Part model, mm, in its own coordinate system. A direction names the side the tool comes from. Coordinates: 2 decimals unless noted, no trailing zeros. Write each loop counter-clockwise with the first axis right and the second up, starting at its lowest first coordinate (ties: lowest second). Pieces come first, ordered by that corner, then holes. Notation, with made-up numbers: M 38,16 L 79,16 A29 cw 79,46 Z; hole C 44,26.5 d3. An arc over 180 degrees is marked long. Use a Markdown table: item, result. Add a question column.
Q1. Tool access for faces 1 (the flat face through (69, 32, 38)), 2 (the flat face through (69, -38, -32.001)), 3 (the flat face through (4, 30, -6)): list every direction of +Z, -Z, +X, -X, +Y, -Y with a clear straight run to the whole face (end or side of a thin tool).
Q2. Slice it at A-A on y = 15. Write the cut outline in (x, z).
Q3. Slice it at C-C on x = 76. Write the cut outline in (y, z).
Q4. Pin check, flat tips, straight feed: pin 1 Ø4 at (x, y) = (134, -2.5) entering from -Z; pin 2 Ø12 at (x, y) = (73.5, -21.5) entering from +Z. Stop position of each tip, or through.
Q5. Wall check: L1, parallel to Y at x = 2.1, z = -32; L2, parallel to X at y = 37.5, z = -5.5; L3, parallel to Z at x = 38, y = 34.5. Give the ranges that are in metal, low to high. Write a range as from..to.
Q6. Slice it at B-B on z = 0. Write the cut outline in (x, y).
Q7. Mould opens along Z. For faces 4 (the flat face through (69, 36, -34)), 5 (the flat face through (64, -40, -33)), 6 (the flat face through (64, -33, 40)) say: released by +Z, released by -Z, zero draft, split by the parting line, or undercut.
from build123d import *

# Parameters (mm, degrees)
CROQUIS1_W              = 80
CROQUIS1_H              = 80
SALIENTE_EXTRUIR1_DEPTH = 140
CORTAR_EXTRUIR3_DEPTH   = 136
CROQUIS8_R              = 2
CROQUIS8_W              = 55
CROQUIS8_H              = 55
CORTAR_EXTRUIR4_DEPTH   = 136
SALIENTE_EXTRUIR4_DEPTH = 8


with BuildPart() as part:
    # Croquis1 → Saliente-Extruir1 (new body)
    with BuildSketch(Plane.YZ):
        Rectangle(CROQUIS1_W, CROQUIS1_H)
    extrude(amount=SALIENTE_EXTRUIR1_DEPTH)

    # Croquis7 → Cortar-Extruir3 (cut)
    with BuildSketch(Plane.YZ.offset(140)):
        Polygon((-40, 32.000605379), (-36, 32.000605379), (-36, 36), (-32, 36), (-32, 40), (32, 40), (32, 36), (36, 36), (36, 32.000605379), (40, 32.000605379), (40, -32.000605379), (36, -32.000605379), (36, -36), (32, -36), (32, -40), (-32, -40), (-32, -36), (-36, -36), (-36, -32.000605379), (-40, -32.000605379), align=None)
    extrude(amount=-CORTAR_EXTRUIR3_DEPTH, mode=Mode.SUBTRACT)

    # Croquis8 → Cortar-Extruir4 (cut)
    with BuildSketch(Plane.YZ.offset(4)):
        with Locations(Location((-32, 32, 0), (0, 0, 270))):
            Circle(CROQUIS8_R)
        with Locations(Location((-32, -32, 0), (0, 0, 270))):
            Circle(CROQUIS8_R)
        with Locations(Location((32, -32, 0), (0, 0, 270))):
            Circle(CROQUIS8_R)
        with Locations(Location((32, 32, 0), (0, 0, 270))):
            Circle(CROQUIS8_R)
        Rectangle(CROQUIS8_W, CROQUIS8_H)
    extrude(amount=-CORTAR_EXTRUIR4_DEPTH, mode=Mode.SUBTRACT)

    # Croquis9 → Saliente-Extruir4 (add)
    with BuildSketch(Plane.YZ.offset(140)):
        Polygon((32, -40), (40, -40), (40, 40), (-40, 40), (-40, -40), (-32, -40), (-32, 32), (32, 32), align=None)
    extrude(amount=-SALIENTE_EXTRUIR4_DEPTH)


solid = part.part
Recorded:
| question | item | result |
|---|---|---|
| 1 | face 1 | +Z, -Z |
| 1 | face 2 | +Y, -Y |
| 1 | face 3 | none |
| 2 | outline | M 0,-40 L 4,-40 L 4,-27.5 L 0,-27.5 Z; M 0,27.5 L 4,27.5 L 4,40 L 0,40 Z; M 132,32 L 140,32 L 140,40 L 132,40 Z |
| 3 | outline | M -40,-40 L -32,-40 L -32,-36 L -36,-36 L -36,-32 L -40,-32 Z; M -40,32 L -36,32 L -36,36 L -32,36 L -32,40 L -40,40 Z; M 32,-40 L 40,-40 L 40,-32 L 36,-32 L 36,-36 L 32,-36 Z; M 32,36 L 36,36 L 36,32 L 40,32 L 40,40 L 32,40 Z |
| 4 | pin 1 | z = 32 |
| 4 | pin 2 | through |
| 5 | L1 | -40..-34, -30..30, 34..40 |
| 5 | L2 | 0..4, 132..140 |
| 5 | L3 | -40..-36, 36..40 |
| 6 | outline | M 0,-40 L 4,-40 L 4,-27.5 L 0,-27.5 Z; M 0,27.5 L 4,27.5 L 4,40 L 0,40 Z; M 132,-40 L 140,-40 L 140,-32 L 132,-32 Z; M 132,32 L 140,32 L 140,40 L 132,40 Z |
| 7 | face 4 | undercut |
| 7 | face 5 | zero draft |
| 7 | face 6 | released by +Z |
